from build123d import *

# Parameters (mm, degrees)
SKETCH2_W              = 132
SKETCH2_H              = 75
BOSS_EXTRUDE1_DEPTH    = 5.461
F_8_CLEARANCE_HOLE1_D  = 4.4958
F_10_CLEARANCE_HOLE1_D = 5.1054
FILLET1_R              = 5
SKETCH7_W              = 69.27
SKETCH7_H              = 31
CUT_EXTRUDE1_DEPTH     = 6.461


with BuildPart() as part:
    # Sketch2 → Boss-Extrude1 (new body)
    with BuildSketch(Plane(origin=(0, 0, 0), x_dir=(1, 0, 0), z_dir=(0, 1, 0))):
        Rectangle(SKETCH2_W, SKETCH2_H)
    extrude(amount=BOSS_EXTRUDE1_DEPTH)

    # #8 Clearance Hole1 (through all)
    with Locations(Plane(origin=(0, 5.461, 0), x_dir=(1, 0, 0), z_dir=(0, 1, 0))):
        with Locations((46, -31), (-46, 31), (-46, -31), (46, 31)):
            Hole(F_8_CLEARANCE_HOLE1_D / 2)

    # #10 Clearance Hole1 (through all)
    with Locations(Plane(origin=(0, 5.461, 0), x_dir=(1, 0, 0), z_dir=(0, 1, 0))):
        with Locations((60.325, -31.75), (-60.325, 31.75), (-60.325, -31.75), (60.325, 31.75)):
            Hole(F_10_CLEARANCE_HOLE1_D / 2)

    # Fillet1
    fillet1_edges = [part.edges().sort_by_distance(p)[0] for p in [
        (66, 2.7305, 37.5),
        (-66, 2.7305, 37.5),
        (-66, 2.7305, -37.5),
        (66, 2.7305, -37.5),
    ]]
    fillet(fillet1_edges, radius=FILLET1_R)

    # Sketch7 → Cut-Extrude1 (cut, through all)
    with BuildSketch(Plane(origin=(0, 5.461, 0), x_dir=(1, 0, 0), z_dir=(0, 1, 0))):
        with Locations((-0.765, 0)):
            Rectangle(SKETCH7_W, SKETCH7_H)
    extrude(amount=-CUT_EXTRUDE1_DEPTH, mode=Mode.SUBTRACT)


solid = part.part
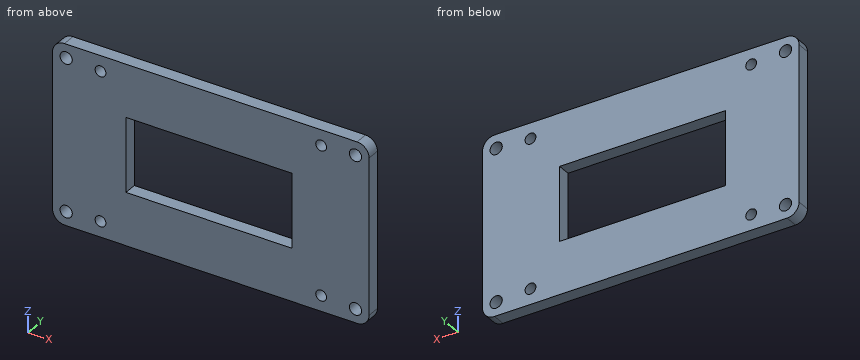
Work out the finished part from the listing and answer in its coordinate system (mm). Coordinates: 2 decimals unless noted, no trailing zeros. Loops run counter-clockwise (first coordinate to the right, second up) from the corner with the lowest first, then second, coordinate; pieces in that order, holes last. Notation, with made-up numbers: M 2,49.5 L 47,49.5 A21 cw 47,82.5 Z; hole C 33.5,51.25 d9. An arc over 180 degrees is marked long. Answer in a Markdown table with one row per item. Add a question column.
1. Find section A-A, the plane x = -46. Write down the section's boundary in (y, z), then the cut area to 3 significant figures.
2. Find section D-D, the plane y = 2.55. State how many separate pieces and enclosed holes the cut face has, then the cut area to 3 significant figures.
3. Find section C-C, the plane z = 6.5. Write down the section's boundary in (x, y), then the cut area to 3 significant figures.
4. Find section B-B, the plane x = 15.5. Write down the section's boundary in (y, z).
5. Flat-ended cylindrical pins translate along their axes: P1, Ø2.5, axis at x = 46, z = -31, coming from the -Y side; P2, Ø6, axis at x = -60.325, z = -31.75, coming from the +Y side. Find the tip coordinate at first contact, or state that the pin passes through.
6. Consider L1, parallel to Z at x = -0.5, y = 4.1; L2, parallel to Z at x = -46, y = 2.05; L3, parallel to X at y = 2.15, z = -32.5. Determine where each line is inside the solid, lowest interval first.
Reported:
| question | item | result |
|---|---|---|
| 1 | outline | M 0,-37.5 L 5.46,-37.5 L 5.46,-33.25 L 0,-33.25 Z; M 0,-28.75 L 5.46,-28.75 L 5.46,28.75 L 0,28.75 Z; M 0,33.25 L 5.46,33.25 L 5.46,37.5 L 0,37.5 Z |
| 1 | area | 360 mm^2 |
| 2 | separate pieces | 1 |
| 2 | enclosed holes | 9 |
| 2 | area | 7,590 mm^2 |
| 3 | outline | M -66,0 L -35.4,0 L -35.4,5.46 L -66,5.46 Z; M 33.87,0 L 66,0 L 66,5.46 L 33.87,5.46 Z |
| 3 | area | 343 mm^2 |
| 4 | outline | M 0,-37.5 L 5.46,-37.5 L 5.46,-15.5 L 0,-15.5 Z; M 0,15.5 L 5.46,15.5 L 5.46,37.5 L 0,37.5 Z |
| 5 | P1 | passes through |
| 5 | P2 | stops at y = 5.46 |
| 6 | L1 | z = -37.5 to -15.5, 15.5 to 37.5 |
| 6 | L2 | z = -37.5 to -33.25, -28.75 to 28.75, 33.25 to 37.5 |
| 6 | L3 | x = -66 to -62.77, -57.88 to -47.67, -44.33 to 44.33, 47.67 to 57.88, 62.77 to 66 |
